Build history of the part. All positions in model axes, mm. Face numbers are marked on the shaded views. A direction names the side the tool comes from. Round coordinates to 2 decimals unless told otherwise and drop trailing zeros. Write each loop counter-clockwise with the first axis right and the second up, starting at its lowest first coordinate (ties: lowest second). Pieces come first, ordered by that corner, then holes.
Item 1: Mould opens along Y. For the marked faces 1, 2 and 3 say: +Y half, -Y half, draft (parallel to the pull), parting line (faces both ways), or undercut.
Item 2: Wall check: probe 1 along X at (y, z) = (2.25, -1.3); probe 2 along Z at (x, y) = (1.5, 1.65); probe 3 along Z at (x, y) = (13.75, -0.65). Give the ranges that are in metal, low to high.
Item 3: Band-saw the part on A-A, the plane x = 1. Write the cut outline in (y, z).
Item 4: 3-axis set-ups, long thin cutter, end or side, ignore diameter. For the marked faces 4, 5 and 6: which of +Z, -Z, +X, -X, +Y, -Y reach the whole face in a straight line?
Item 5: Drop flat-ended pins along their axis: pin 1 Ø1.5 at (y, z) = (1.5, -2) entering from +X; pin 2 Ø1 at (x, y) = (7.5, 0.5) entering from -Z; pin 3 Ø0.5 at (y, z) = (0.5, 1) entering from -X. Give the stop position or say it passes through.
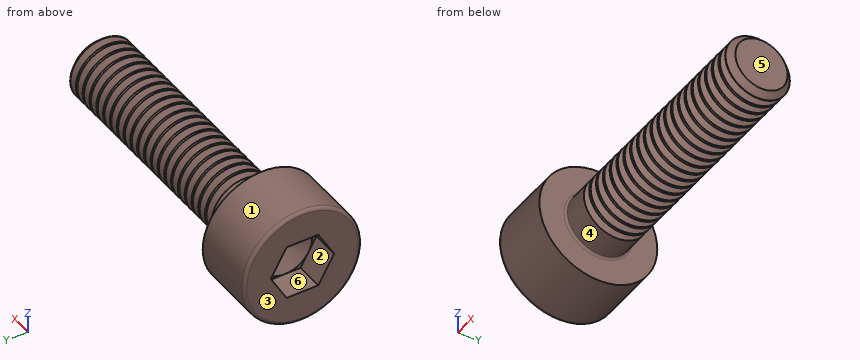
```python
from build123d import *

# Parameters (mm, degrees)
FILLET1_R       = 0.1
FILLET2_R       = 0.15
HEX_2_DEPTH     = 1.3
THDSCHPAT_COUNT = 21
THDSCHPAT_PITCH = 0.5


with BuildPart() as part:
    # BodySke → Base-Revolve (revolve)
    with BuildSketch(Plane.XY):
        Polygon((0, 0), (0, 2.75), (3, 2.75), (3, 1.5), (14.7195, 1.5), (15, 1.2195), (15, 0), align=None)
    revolve(axis=Axis((-31.75, 0, 0), (1, 0, 0)))

    # Fillet1
    fillet1_edges = [part.edges().sort_by_distance(p)[0] for p in [
        (3, -1.5, 0),
    ]]
    fillet(fillet1_edges, radius=FILLET1_R)

    # Fillet2
    fillet2_edges = [part.edges().sort_by_distance(p)[0] for p in [
        (0, -2.75, 0),
    ]]
    fillet(fillet2_edges, radius=FILLET2_R)

    # Sketch2 → Hex-PreBroach (revolve, cut)
    with BuildSketch(Plane.XY):
        Polygon((0, 1.28), (1.3, 1.28), (2.039008345, 0), (0, 0), align=None)
    revolve(axis=Axis((0, 0, 0), (1, 0, 0)), mode=Mode.SUBTRACT)

    # Sketch3 → Hex 2 (cut)
    with BuildSketch(Plane(origin=(0, 0, 0), x_dir=(0, 0.5, 0.866025404), z_dir=(-1, 0, 0))):
        Polygon((0.739008345, 1.28), (-0.739008345, 1.28), (-1.478016689, 0), (-0.739008345, -1.28), (0.739008345, -1.28), (1.478016689, 0), align=None)
    extrude(amount=-HEX_2_DEPTH, mode=Mode.SUBTRACT)

    # ThdSchSke → ThreadSchematic (revolve, cut)
    with BuildSketch(Plane.XY):
        Polygon((4.5, -1.2195), (4.303591786, -1.5), (4.303591786, -1.875), (4.696408214, -1.875), (4.696408214, -1.5), align=None)
    threadschematic = revolve(axis=Axis((-3.175, 0, 0), (1, 0, 0)), mode=Mode.SUBTRACT)

    # ThdSchPat: ThreadSchematic ×21
    with Locations(*[(i * THDSCHPAT_PITCH, 0, 0) for i in range(1, THDSCHPAT_COUNT)]):
        add(threadschematic, mode=Mode.SUBTRACT)


solid = part.part
```
Results:
1. face 1: parting line
1. face 2: undercut
1. face 3: draft
2. probe 1: x = 0 to 3
2. probe 2: z = -2.2 to 2.2
2. probe 3: z = -1.35 to 1.35
3. outline: circle Ø5.5 at (0, 0); hole (-1.48, 0) - (-0.74, -1.28) - (0.74, -1.28) - (1.48, 0) - (0.74, 1.28) - (-0.74, 1.28) - close
4. face 4: +X
4. face 5: +Z, -Z, +X, +Y, -Y
4. face 6: -X
5. pin 1: stops at x = 3
5. pin 2: stops at z = -1.5
5. pin 3: stops at x = 1.3
